Could you check a few things on this model? Use its own coordinates, in mm. Give positions to 0.01 mm unless a question says otherwise; leave off trailing zeros. Loops run counter-clockwise (first coordinate to the right, second up) from the corner with the lowest first, then second, coordinate; pieces in that order, holes last. Notation, with made-up numbers: (-32, 11.25) - (-8, 11.25) arc R14 cw to (-8, 30.25) - close; hole circle Ø10 at (87.25, -8). An arc over 180 degrees is marked (long way). Use CSV: the item, a comma, the result in double quotes.
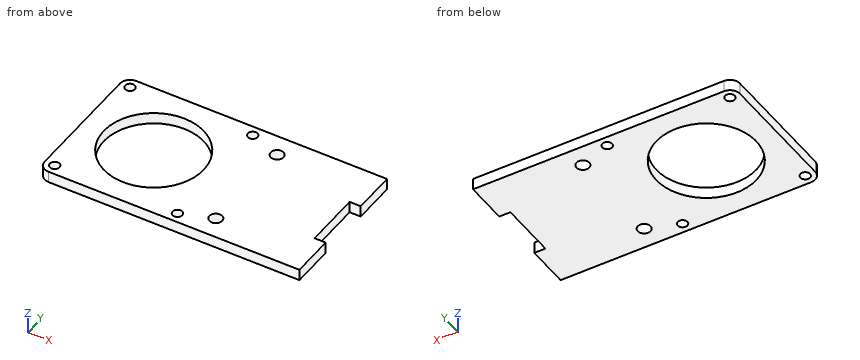
from build123d import *

# Parameters (mm, degrees)
SKETCH_1_W         = 50
SKETCH_1_H         = 87.5
SKETCH_1_R         = 17.5
SKETCH_1_W_2       = 15
SKETCH_1_H_2       = 3.9
EXTRUDE_1_DEPTH    = 4
HOLE_WIZARD_M3_1_D = 3.4
HOLE_WIZARD_M4_1_D = 4.5
FILLET_2_R         = 3.5


with BuildPart() as part:
    # Sketch 1 → Extrude 1 (new body)
    with BuildSketch(Plane(origin=(0, 0, 0), x_dir=(0, 1, 0), z_dir=(0, 0, 1))):
        with Locations((25, 43.75)):
            Rectangle(SKETCH_1_W, SKETCH_1_H)
        with Locations((25, 62.5)):
            Circle(SKETCH_1_R, mode=Mode.SUBTRACT)
        with Locations((42.5, -1.95)):
            Rectangle(SKETCH_1_W_2, SKETCH_1_H_2)
        with Locations((7.5, -1.95)):
            Rectangle(SKETCH_1_W_2, SKETCH_1_H_2)
    extrude(amount=EXTRUDE_1_DEPTH)

    # Hole Wizard M3 _1 (through all)
    with Locations(Plane.XY.offset(4)):
        with Locations((-84, 3.5), (-84, 46.5), (-41, 46.5), (-41, 3.5)):
            Hole(HOLE_WIZARD_M3_1_D / 2)

    # Hole Wizard M4 _1 (through all)
    with Locations(Plane.XY.offset(4)):
        with Locations((-30, 42.5), (-30, 7.5)):
            Hole(HOLE_WIZARD_M4_1_D / 2)

    # Fillet 2
    fillet_2_edges = [part.edges().sort_by_distance(p)[0] for p in [
        (-87.5, 0, 2),
        (-87.5, 50, 2),
    ]]
    fillet(fillet_2_edges, radius=FILLET_2_R)


solid = part.part
1) Suppose I cut it at A-A (y = 25). Please give me the cut outline in (x, z).
Answer below:
outline,"(-87.5, 0) - (-80, 0) - (-80, 4) - (-87.5, 4) - close; (-45, 0) - (0, 0) - (0, 4) - (-45, 4) - close"
2) Suppose I cut it at C-C (x = -56). Please give me the cut outline in (y, z), plus the area to 3 significant figures.
Answer below:
outline,"(0, 0) - (8.75, 0) - (8.75, 4) - (0, 4) - close; (41.25, 0) - (50, 0) - (50, 4) - (41.25, 4) - close"
area,"70.0 mm2"
3) Suppose I cut it at B-B (z = 2.9). Please give me the cut outline in (x, y), plus the area to 3 significant figures.
Answer below:
outline,"(-87.5, 3.5) arc R3.5 ccw to (-84, 0) - (3.9, 0) - (3.9, 15) - (0, 15) - (0, 35) - (3.9, 35) - (3.9, 50) - (-84, 50) arc R3.5 ccw to (-87.5, 46.5) - close; hole circle Ø3.4 at (-84, 3.5); hole circle Ø3.4 at (-84, 46.5); hole circle Ø35 at (-62.5, 25); hole circle Ø3.4 at (-41, 3.5); hole circle Ø3.4 at (-41, 46.5); hole circle Ø4.5 at (-30, 7.5); hole circle Ø4.5 at (-30, 42.5)"
area,"3,460 mm2"
4) I need wall thicknesses on line 1 along Y through (x, z) = (-30, 2.3); line 2 along Y through (x, z) = (-84, 1.65); line 3 along X through (y, z) = (25, 2.9). Which ranges of each line are inside material? Lowest first, please.
Answer below:
line 1,"y = 0 to 5.25, 9.75 to 40.25, 44.75 to 50"
line 2,"y = 0 to 1.8, 5.2 to 44.8, 48.2 to 50"
line 3,"x = -87.5 to -80, -45 to 0"
5) I'm going to push flat-ended pins straight in: P1, Ø2.5, axis at x = -30, y = 7.5, coming from the -Z side; P2, Ø1.5, axis at y = 16, z = 1.5, coming from the +X side. Where does each tip first touch, or does it pass through?
Answer below:
P1,"passes through"
P2,"stops at x = 0"
